Check sheet for the drawn part. Datum: minimum x, y, z corner. Units: mm. A direction names the side the tool comes from. Round coordinates to 2 decimals unless told otherwise and drop trailing zeros. Write each loop counter-clockwise with the first axis right and the second up, starting at its lowest first coordinate (ties: lowest second). Pieces come first, ordered by that corner, then holes.
Item 1: Cross-section at A-A on x = 5. Enter the section's corners in (y, z).
Item 2: Material ranges on line 1 (Y direction, x = 5, z = 9); line 2 (X direction, y = 13, z = 5.25); line 3 (Z direction, x = 8.5, y = 26), recorded low to high.
Item 3: Cross-section at B-B on z = 5. Enter the section's corners in (x, y), plus the area to 3 significant figures.
Item 4: Cross-section at D-D on x = 0.75. Enter the section's corners in (y, z), plus the area to 3 significant figures.
Item 5: Go/stop test with flat-tipped pins: pin 1 Ø5 at (x, y) = (8.5, 23.5) entering from -Z; pin 2 Ø2 at (x, y) = (8.5, 9) entering from +Z; pin 3 Ø2 at (y, z) = (14, 6.5) entering from +X. Record where each tip stops, or that it passes through.
Item 6: Cross-section at C-C on y = 8. Enter the section's corners in (x, z).
Item 7: Tool access check on the marked faces 1, 2 and 3. Record the directions out of +Z, -Z, +X, -X, +Y, -Y that give a thin tool (end or side, any length) a straight path to the whole face; none if there is none.
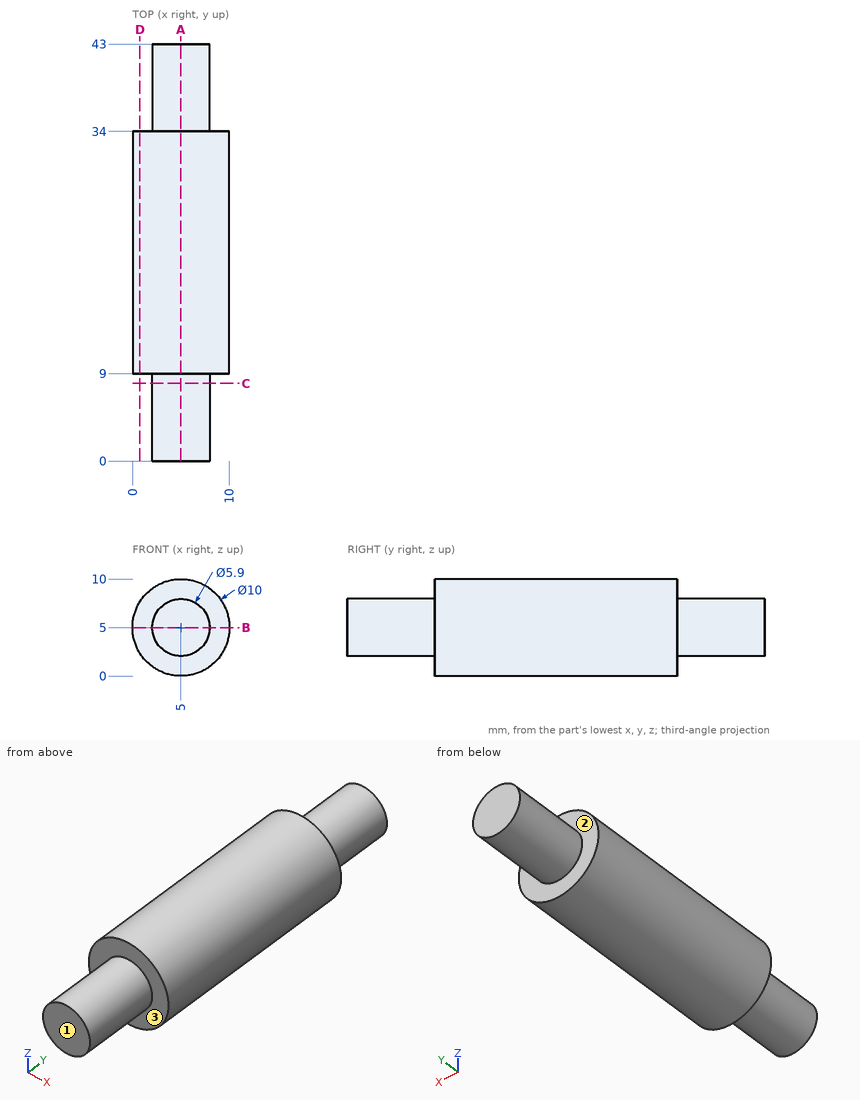
Response values:
1. outline: (0, 2.05) - (9, 2.05) - (9, 0) - (34, 0) - (34, 2.05) - (43, 2.05) - (43, 7.95) - (34, 7.95) - (34, 10) - (9, 10) - (9, 7.95) - (0, 7.95) - close
2. line 1: y = 9 to 34
2. line 2: x = 0.01 to 9.99
2. line 3: z = 1.43 to 8.57
3. outline: (0, 9) - (2.05, 9) - (2.05, 0) - (7.95, 0) - (7.95, 9) - (10, 9) - (10, 34) - (7.95, 34) - (7.95, 43) - (2.05, 43) - (2.05, 34) - (0, 34) - close
3. area: 356 mm2
4. outline: (9, 2.37) - (34, 2.37) - (34, 7.63) - (9, 7.63) - close
4. area: 132 mm2
5. pin 1: stops at z = 0.1
5. pin 2: stops at z = 9.33
5. pin 3: stops at x = 9.97
6. outline: circle Ø5.9 at (5, 5)
7. face 1: +Z, -Z, +X, -X, -Y
7. face 2: +Y
7. face 3: -Y
